from build123d import *

# Parameters (mm, degrees)
SKETCH1_R           = 13.25
SKETCH1_R_2         = 5
SKETCH1_R_3         = 1.55
SKETCH1_R_4         = 4
BOSS_EXTRUDE1_DEPTH = 14.8
SKETCH1_3_R         = 6
SKETCH1_3_R_2       = 5
EXTRUDE_THIN1_DEPTH = 15.8


with BuildPart() as part:
    # Sketch1 → Boss-Extrude1 (new, symmetric)
    # profile 1 of 2: a face of its own
    with BuildSketch(Plane.XY):
        Circle(SKETCH1_R)
        Circle(SKETCH1_R_2, mode=Mode.SUBTRACT)
        with Locations((-8.660254038, -5)):
            Circle(SKETCH1_R_3, mode=Mode.SUBTRACT)
        with Locations((8.660254038, -5)):
            Circle(SKETCH1_R_3, mode=Mode.SUBTRACT)
        with Locations((0, 10)):
            Circle(SKETCH1_R_3, mode=Mode.SUBTRACT)
    # profile 2 of 2: a face of its own
    with BuildSketch(Plane.XY):
        Circle(SKETCH1_R_2)
        Circle(SKETCH1_R_4, mode=Mode.SUBTRACT)
    extrude(amount=BOSS_EXTRUDE1_DEPTH, both=True)

    # Sketch1_3 → Extrude-Thin1 (add, symmetric)
    with BuildSketch(Plane.XY):
        Circle(SKETCH1_3_R)
        Circle(SKETCH1_3_R_2, mode=Mode.SUBTRACT)
    extrude(amount=EXTRUDE_THIN1_DEPTH, both=True)


solid = part.part
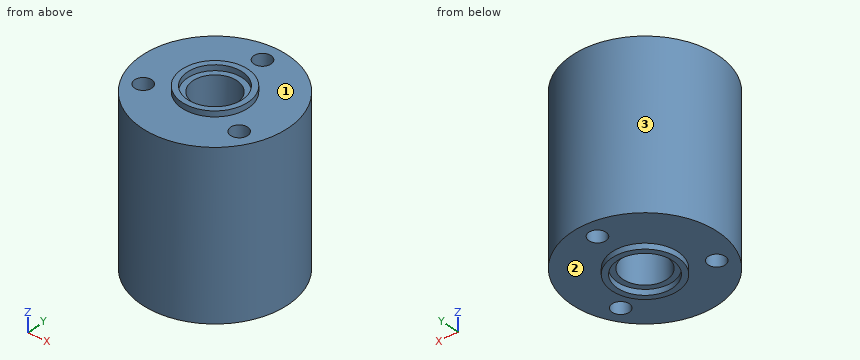
For this review, take the finished solid that the model builds, in its own axes (mm). Face numbers are marked on the shaded views. A direction names the side the tool comes from. Round coordinates to 2 decimals unless told otherwise and drop trailing zeros. Order: outer loops, then holes, each group sorted by start corner. A loop starts at its lowest first (then second) coordinate and runs counter-clockwise, first axis right, second up. Notation, with made-up numbers: (-11.5, 28.25) -> (-0.5, 28.25) arc R11 ccw to (-0.5, 46.25) -> close; hole circle Ø2 at (86.25, -17.75). An arc over 180 degrees is marked (long way). Write item = value, one per line. Start each with the question number.
1) Take a section at B-B on x = 0. State the section outline as (y, z) points.
2) Take a section at A-A on y = 0. State the section outline as (x, z) points.
3) To check wall thickness, follow line 1 (Y direction, x = 0, z = 14.5); line 2 (Z direction, x = -4.25, y = -8.5); line 3 (Y direction, x = 10, z = 4.5). State the ranges of each line that lie inside material, in increasing order. Write a range as from..to.
4) Take a section at D-D on x = 9.5. State the section outline as (y, z) points.
5) Take a section at C-C on z = -12.5. State the section outline as (x, y) points, plus the area to 3 significant figures.
6) Tool access review of the marked faces 1, 2 and 3: name each direction out of +Z, -Z, +X, -X, +Y, -Y from which nothing blocks a thin tool from reaching the whole face with its end or side.
7) Insertion check: pin 1 (3 mm diameter, centred on x = -8, z = 11.5, fed in from +Y); pin 2 (10 mm diameter, centred on y = 6.5, z = 10.5, fed in from -X); pin 3 (8 mm diameter, centred on x = 0, y = 2, fed in from -Z); pin 4 (2 mm diameter, centred on x = 6.5, y = 7.5, fed in from -Z). Each pin has a flat end and moves straight along its axis. Give the tip position at first contact, or say it passes through.
Verdict:
q1.outline = (-13.25, -14.8) -> (-6, -14.8) -> (-6, -15.8) -> (-5, -15.8) -> (-5, -14.8) -> (-4, -14.8) -> (-4, 14.8) -> (-5, 14.8) -> (-5, 15.8) -> (-6, 15.8) -> (-6, 14.8) -> (-13.25, 14.8) -> close; (4, -14.8) -> (5, -14.8) -> (5, -15.8) -> (6, -15.8) -> (6, -14.8) -> (8.45, -14.8) -> (8.45, 14.8) -> (6, 14.8) -> (6, 15.8) -> (5, 15.8) -> (5, 14.8) -> (4, 14.8) -> close; (11.55, -14.8) -> (13.25, -14.8) -> (13.25, 14.8) -> (11.55, 14.8) -> close
q2.outline = (-13.25, -14.8) -> (-6, -14.8) -> (-6, -15.8) -> (-5, -15.8) -> (-5, -14.8) -> (-4, -14.8) -> (-4, 14.8) -> (-5, 14.8) -> (-5, 15.8) -> (-6, 15.8) -> (-6, 14.8) -> (-13.25, 14.8) -> close; (4, -14.8) -> (5, -14.8) -> (5, -15.8) -> (6, -15.8) -> (6, -14.8) -> (13.25, -14.8) -> (13.25, 14.8) -> (6, 14.8) -> (6, 15.8) -> (5, 15.8) -> (5, 14.8) -> (4, 14.8) -> close
q3.line_1 = -13.25..-4, 4..8.45, 11.55..13.25
q3.line_2 = -14.8..14.8
q3.line_3 = -8.69..-5.78, -4.22..8.69
q4.outline = (-9.24, -14.8) -> (-6.3, -14.8) -> (-6.3, 14.8) -> (-9.24, 14.8) -> close; (-3.7, -14.8) -> (9.24, -14.8) -> (9.24, 14.8) -> (-3.7, 14.8) -> close
q5.outline = circle Ø26.5 at (0, 0); hole circle Ø3.1 at (-8.66, -5); hole circle Ø8 at (0, 0); hole circle Ø3.1 at (0, 10); hole circle Ø3.1 at (8.66, -5)
q5.area = 479 mm2
q6.face_1 = +Z
q6.face_2 = -Z
q6.face_3 = +Z, -Z
q7.pin_1 = 11.55
q7.pin_2 = -13.16
q7.pin_3 = -15.8
q7.pin_4 = -14.8
